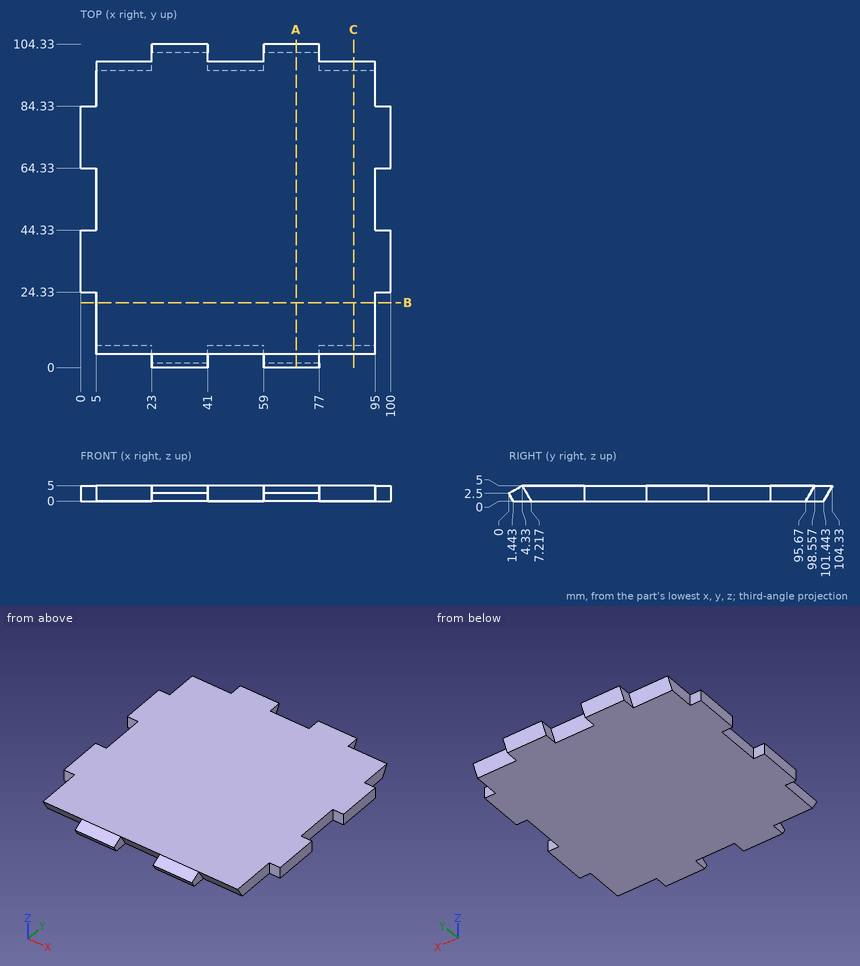
The figure shows three views and two pictorial views of one solid part (mm, origin at its lowest corner). Answer the questions. Coordinates: 2 decimals unless noted, no trailing zeros. Loops run counter-clockwise (first coordinate to the right, second up) from the corner with the lowest first, then second, coordinate; pieces in that order, holes last. Notation, with made-up numbers: M 44.25,-35 L 63.25,-35 A25 cw 63.25,3 Z; hole C -19,-38 d11. An arc over 180 degrees is marked long. Use CSV: the item, a comma, the result in double quotes. Start each with the question number.
(1) Find section A-A, the plane x = 69.5. Give the vertices of the cut face in (y, z).
(2) Find section C-C, the plane x = 88. Give the vertices of the cut face in (y, z), then the cut area to 3 significant figures.
(3) Find section B-B, the plane y = 21. Give the vertices of the cut face in (x, z).
(4) Consider line 1 (X direction, y = 56, z = 0.8); line 2 (Y direction, x = 61, z = 4.1); line 3 (Y direction, x = 47.5, z = 2.2). Determine where each line is inside the solid, lowest interval first.
(5) Given pin 1 Ø2.5 at (y, z) = (12, 2) entering from +X; pin 2 Ø3 at (x, z) = (24, 1) entering from +Y; pin 3 Ø1.5 at (y, z) = (2.5, 2) entering from -X, each flat-ended and moving along its own axis, determine where each tip first touches the part or whether it passes through.
Recorded:
1,outline,"M 0,2.5 L 1.44,0 L 101.44,0 L 104.33,5 L 4.33,5 Z"
2,outline,"M 4.33,5 L 7.22,0 L 95.67,0 L 98.56,5 Z"
2,area,"457 mm^2"
3,outline,"M 5,0 L 95,0 L 95,5 L 5,5 Z"
4,line 1,"x = 5 to 95"
4,line 2,"y = 2.77 to 103.81"
4,line 3,"y = 5.95 to 96.94"
5,pin 1,"stops at x = 95"
5,pin 2,"stops at y = 102.89"
5,pin 3,"stops at x = 23"
